Geometry check sheet. Reference: drawing and pictorial views, mm from the part's lowest x, y, z. Coordinates: 2 decimals unless noted, no trailing zeros. Loops run counter-clockwise (first coordinate to the right, second up) from the corner with the lowest first, then second, coordinate; pieces in that order, holes last. Notation, with made-up numbers: (80.5, 35.25) - (102.5, 35.25) arc R23 ccw to (102.5, 44.25) - close; hole circle Ø6 at (-1.75, 81). An arc over 180 degrees is marked (long way). Use a Markdown table: item, result. Add a question column.
1) Sectioned sample at A-A, the plane x = 33.5. Enter the section's corners in (y, z).
2) Sectioned sample at C-C, the plane x = 6. Enter the section's corners in (y, z), then the cut area to 3 significant figures.
3) Sectioned sample at B-B, the plane y = 1.3. Enter the section's corners in (x, z).
4) Thickness scan on line 1 (X direction, y = 1, z = 25); line 2 (Z direction, x = 33.5, y = 0.5); line 3 (X direction, y = 0.8, z = 2.75). Record the ranges inside material, lowest first.
5) Go/stop test with a flat-tipped pin: P1, Ø1.7, axis at x = 33.5, z = 25, coming from the +Y side. Record where the tip stops, or that it passes through.
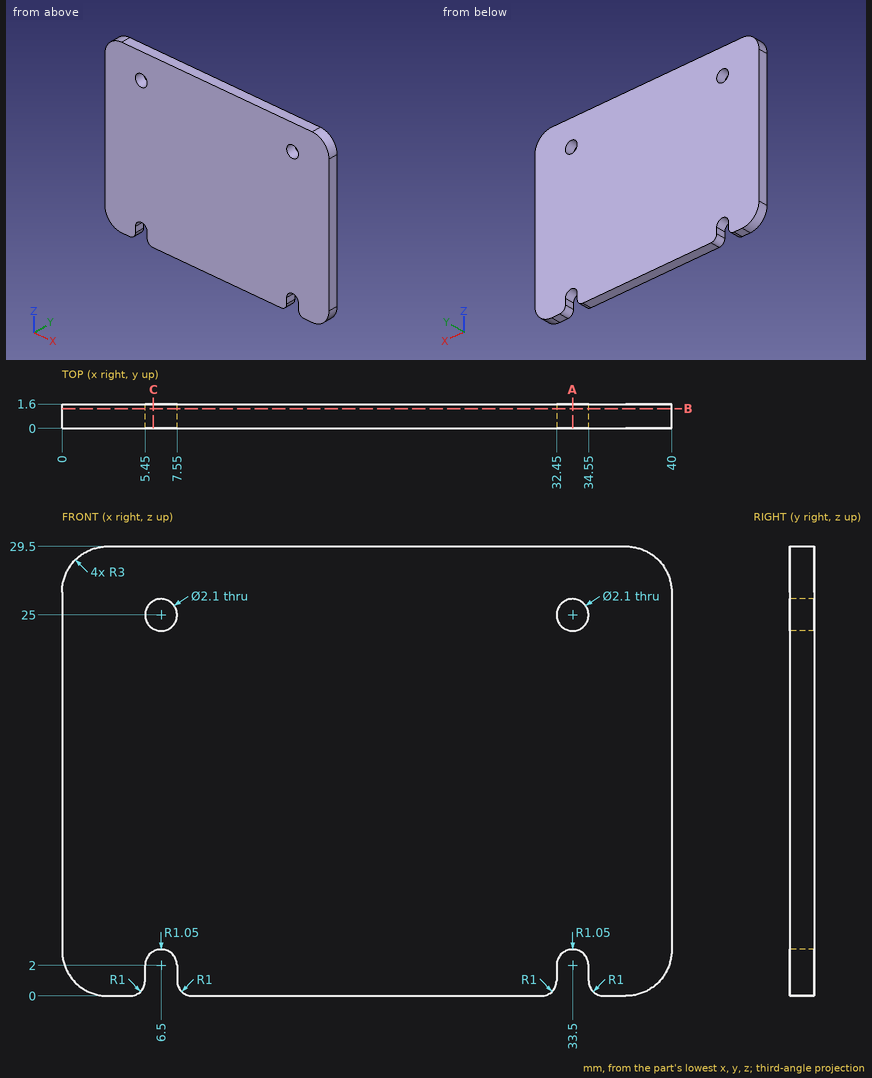
Solved:
| question | item | result |
|---|---|---|
| 1 | outline | (0, 3.05) - (1.6, 3.05) - (1.6, 23.95) - (0, 23.95) - close; (0, 26.05) - (1.6, 26.05) - (1.6, 29.5) - (0, 29.5) - close |
| 2 | outline | (0, 2.92) - (1.6, 2.92) - (1.6, 24.08) - (0, 24.08) - close; (0, 25.92) - (1.6, 25.92) - (1.6, 29.5) - (0, 29.5) - close |
| 2 | area | 39.6 mm2 |
| 3 | outline | (0, 3) arc R3 ccw to (3, 0) - (4.45, 0) arc R1 ccw to (5.45, 1) - (5.45, 2) arc R1.05 cw to (7.55, 2) - (7.55, 1) arc R1 ccw to (8.55, 0) - (31.45, 0) arc R1 ccw to (32.45, 1) - (32.45, 2) arc R1.05 cw to (34.55, 2) - (34.55, 1) arc R1 ccw to (35.55, 0) - (37, 0) arc R3 ccw to (40, 3) - (40, 26.5) arc R3 ccw to (37, 29.5) - (3, 29.5) arc R3 ccw to (0, 26.5) - close; hole circle Ø2.1 at (6.5, 25); hole circle Ø2.1 at (33.5, 25) |
| 4 | line 1 | x = 0 to 5.45, 7.55 to 32.45, 34.55 to 40 |
| 4 | line 2 | z = 3.05 to 23.95, 26.05 to 29.5 |
| 4 | line 3 | x = 0.01 to 5.77, 7.23 to 32.77, 34.23 to 39.99 |
| 5 | P1 | passes through |
